Geometry check sheet. Reference: the model listing, model coordinates, mm. A direction names the side the tool comes from. Coordinates: 2 decimals unless noted, no trailing zeros. Write each loop counter-clockwise with the first axis right and the second up, starting at its lowest first coordinate (ties: lowest second). Pieces come first, ordered by that corner, then holes. Notation, with made-up numbers: (56.5, -8) -> (90.5, -8) arc R16 cw to (90.5, 14) -> close; hole circle Ø2 at (84.5, 57.5). An arc over 180 degrees is marked (long way). Use a Markdown table: item, result.
```python
from build123d import *

# Parameters (mm, degrees)
F1_DEPTH = 25.5
F3_DEPTH = 16.5
F6_D     = 3.5
F7_R     = 8.663852
F7_R_2   = 4.05
F7_R_3   = 9.323293
F8_DEPTH = 40


with BuildPart() as f1:
    # F0 (on Front) → F1 (new body, symmetric)
    with BuildSketch(Plane.XZ):
        with BuildLine():
            Line((-21.26926, 0), (23.73074, 0))
            Line((23.73074, 0), (9.928151, 72.969893))
            ThreePointArc((9.928151, 72.969893), (0, 80.571183), (-9.928151, 72.969893))
            Line((-9.928151, 72.969893), (-21.26926, 0))
        make_face()
    extrude(amount=F1_DEPTH, both=True)


with BuildPart() as f3:
    # F2 (on Front) → F3 (new body, symmetric)
    with BuildSketch(Plane.XZ):
        Polygon((-6.10114, 6), (30, 6), (20, 90), (-30, 90), (-30, 0), (-7.03367, 0), align=None)
    extrude(amount=F3_DEPTH, both=True)


with BuildPart() as f1_1:
    add(f1.part)

    # F4: cut F3
    add(f3.part, mode=Mode.SUBTRACT)

    # F6 (through all)
    with Locations(Plane.XZ.offset(25.5)):
        with Locations((-2, 72), (-15, 4.5)):
            Hole(F6_D / 2)


with BuildPart() as f8:
    # F7 (on Front) → F8 (new body, symmetric)
    with BuildSketch(Plane.XZ):
        with Locations((0, 42.608014)):
            Circle(F7_R)
        with Locations((0, 61.275356)):
            Circle(F7_R_2)
        with Locations((0, 20.42364)):
            Circle(F7_R_3)
    extrude(amount=F8_DEPTH, both=True)


with BuildPart() as f1_2:
    add(f1_1.part)

    # F9: cut F8
    add(f8.part, mode=Mode.SUBTRACT)


solid = f1_2.part
```
Item 1: Section check B-B on z = 55. Record the boundary of the cut face in (x, y).
Answer block:
| item | result |
|---|---|
| outline | (-12.72, -25.5) -> (13.33, -25.5) -> (13.33, -16.5) -> (-12.72, -16.5) -> close; (-12.72, 16.5) -> (13.33, 16.5) -> (13.33, 25.5) -> (-12.72, 25.5) -> close |
Item 2: Section check A-A on x = -18. Record the boundary of the cut face in (y, z).
Answer block:
| item | result |
|---|---|
| outline | (-25.5, 0) -> (-16.5, 0) -> (-16.5, 21.03) -> (-25.5, 21.03) -> close; (16.5, 0) -> (25.5, 0) -> (25.5, 21.03) -> (16.5, 21.03) -> close |
Item 3: Mould release check, pull along Z, two halves, no side actions. Record for faces 1 (the flat face through (-6.574, -0.231, 2.958)), 2 (the flat face through (1, 25.5, 32)), 3 (the cylindrical face through (4.66, 20.94, 49.91)): +Z half, -Z half, draft (parallel to the pull), parting line (faces both ways), or undercut.
Answer block:
| item | result |
|---|---|
| face 1 | +Z half |
| face 2 | draft |
| face 3 | undercut |
Item 4: Thickness scan on L1, parallel to Z at x = 0, y = -18; L2, parallel to Y at x = -14, z = 32; L3, parallel to Z at x = -2, y = -19. Record the ranges inside material, lowest first. Write a range as [from, to].
Answer block:
| item | result |
|---|---|
| L1 | z = [0, 11.1], [29.75, 33.94], [51.27, 57.23], [65.33, 80.57] |
| L2 | y = [-25.5, -16.5], [16.5, 25.5] |
| L3 | z = [0, 11.32], [29.53, 34.18], [51.04, 57.75], [64.8, 70.25], [73.75, 80.37] |
Item 5: Section check D-D on y = 21.5. Record the boundary of the cut face in (x, z).
Answer block:
| item | result |
|---|---|
| outline | (-21.27, 0) -> (23.73, 0) -> (9.93, 72.97) arc R10.28 ccw to (-9.93, 72.97) -> close; hole circle Ø3.5 at (-15, 4.5); hole circle Ø18.65 at (0, 20.42); hole circle Ø17.33 at (0, 42.61); hole circle Ø8.1 at (0, 61.28); hole circle Ø3.5 at (-2, 72) |
Item 6: Tool access check on faces 4 (the cylindrical face through (0.19, 20.94, 80.57)), 5 (the flat face through (8, 0, 6)). Record the directions out of +Z, -Z, +X, -X, +Y, -Y that give a thin tool (end or side, any length) a straight path to the whole face; none if there is none.
Answer block:
| item | result |
|---|---|
| face 4 | +Z, +Y, -Y |
| face 5 | +Z, +X, -X |
Item 7: Section check C-C on z = 4.5. Record the boundary of the cut face in (x, y), then the cut area to 3 significant figures.
Answer block:
| item | result |
|---|---|
| outline | (-20.57, -25.5) -> (-16.75, -25.5) -> (-16.75, -16.5) -> (-20.57, -16.5) -> close; (-20.57, 16.5) -> (-16.75, 16.5) -> (-16.75, 25.5) -> (-20.57, 25.5) -> close; (-13.25, -25.5) -> (22.88, -25.5) -> (22.88, 25.5) -> (-13.25, 25.5) -> (-13.25, 16.5) -> (-6.33, 16.5) -> (-6.33, -16.5) -> (-13.25, -16.5) -> close |
| area | 1,680 mm^2 |
Item 8: Depth check by flat-ended pin: P1, Ø20, axis at x = 0, z = 42.61, coming from the +Y side; P2, Ø12, axis at x = -14.5, y = 13.5, coming from the +Z side; P3, Ø8.5, axis at x = 13, y = 2.5, coming from the +Z side; P4, Ø8, axis at y = 13.5, z = 53, coming from the +X side. Enter the tip coordinate at first touch or a pass-through.
Answer block:
| item | result |
|---|---|
| P1 | stops at y = 25.5 |
| P2 | stops at z = 74.67 |
| P3 | stops at z = 6 |
| P4 | stops at x = 14.21 |
